Input: part model. Units: mm. Frame: model coordinates. A direction names the side the tool comes from. Coordinates: 2 decimals unless noted, no trailing zeros. Loops run counter-clockwise (first coordinate to the right, second up) from the corner with the lowest first, then second, coordinate; pieces in that order, holes last.
```python
from build123d import *

# Parameters (mm, degrees)
MAIN_DEPTH    = 12.7
SKETCH2_R     = 7.9375
AXLE_DEPTH    = 12.7
SKETCH5_W     = 12.7
SKETCH5_H     = 25.4
BARWIDE_DEPTH = 12.7


with BuildPart() as part:
    # Sketch1 → main (new body)
    with BuildSketch(Plane(origin=(0, 0, 0), x_dir=(0, 0, -1), z_dir=(1, 0, 0))):
        with BuildLine():
            Line((0, 31.75), (50.8, 31.75))
            Line((50.8, 31.75), (184.15, -139.7))
            Line((184.15, -139.7), (196.85, -139.7))
            Line((196.85, -139.7), (196.85, -152.4))
            Line((196.85, -152.4), (209.55, -152.4))
            Line((209.55, -152.4), (209.55, -139.7))
            Line((209.55, -139.7), (311.15, -165.1))
            Line((311.15, -165.1), (184.15, -165.1))
            Line((184.15, -165.1), (50.8, -31.75))
            Line((50.8, -31.75), (0, -31.75))
            ThreePointArc((0, -31.75), (-31.75, 0), (0, 31.75))
        make_face()
    extrude(amount=MAIN_DEPTH)

    # Sketch2 → axle (cut)
    with BuildSketch(Plane(origin=(12.7, 0, 0), x_dir=(0, 0, -1), z_dir=(1, 0, 0))):
        Circle(SKETCH2_R)
    extrude(amount=-AXLE_DEPTH, mode=Mode.SUBTRACT)

    # Sketch5 → barwide (cut)
    with BuildSketch(Plane(origin=(0, 36.585769231, -47.038846154), x_dir=(-1, 0, 0), z_dir=(0, 0.6139406135149222, -0.789352217376325))):
        with Locations((-6.35, -109.029668746)):
            Rectangle(SKETCH5_W, SKETCH5_H)
    extrude(amount=-BARWIDE_DEPTH, mode=Mode.SUBTRACT)


solid = part.part
```
Item 1: Mould query, pull axis Y, two halves, no side actions, for faces 1 (the face through (6, -165.1, -249)), 2 (the face through (6.261, -0.698, 31.742)), 3 (the face through (6.44, -57.13, -103.84)). Classes: +Y half, -Y half, draft (parallel to the pull), parting line (faces both ways), or undercut.
Result:
face 1: -Y half
face 2: parting line
face 3: undercut
Item 2: Line query: L1, parallel to Y at x = 12, z = -201.5; L2, parallel to Z at x = 12, y = -43; L3, parallel to Y at x = 8, z = -228. Output: solid intervals per line, ascending.
Result:
L1: y = -165.1 to -152.4
L2: z = -101.62 to -62.05
L3: y = -165.1 to -144.31
Item 3: Section query C-C (y = -20). Output: boundary loops of the cut face in (x, z).
Result:
outline: (0, -91.05) - (12.7, -91.05) - (12.7, 24.66) - (0, 24.66) - close
Item 4: Section query A-A (y = 0). Output: boundary loops of the cut face in (x, z).
Result:
outline: (0, -75.49) - (12.7, -75.49) - (12.7, -7.94) - (0, -7.94) - close; (0, 7.94) - (12.7, 7.94) - (12.7, 31.75) - (0, 31.75) - close
Item 5: Contact query for flat-ended pins moving along their axis: P1, Ø1.5, axis at x = 3.5, y = -79.5, coming from the -Z side; P2, Ø20.5, axis at y = 0, z = 0, coming from the +X side; P3, Ø4, axis at x = 6, z = -202.5, coming from the +Y side; P4, Ø5, axis at x = 8.5, y = 2, coming from the +Z side. Output: stop coordinate, or through.
Result:
P1: stops at z = -137.91
P2: stops at x = 12.7
P3: stops at y = -152.4
P4: stops at z = 31.75
Item 6: Reachability of faces 4 (the face through (6, -31.75, -26)), 5 (the face through (6, -139.7, -190)), 6 (the face through (6, -152.4, -203)), 7 (the face through (6.44, -7.75, 1.72)), 8 (the face through (6.439, -43.296, -101.237)) from +Z, -Z, +X, -X, +Y, -Y: full face, straight path, thin tool, end or side. Return the list, or none.
Result:
face 4: +Z, +X, -X, -Y
face 5: -Z, +X, -X, +Y
face 6: +X, -X, +Y
face 7: +X, -X
face 8: -Z, +X, -X
Item 7: Section query B-B (z = -81). Output: boundary loops of the cut face in (x, y).
Result:
outline: (0, -61.95) - (12.7, -61.95) - (12.7, -7.08) - (0, -7.08) - close
